from build123d import *

# Parameters (mm, degrees)
F0_W      = 5
F0_H      = 37.2
F0_W_2    = 20
F0_H_2    = 20
F0_W_3    = 23.5
F0_H_3    = 32.2
F0_R      = 10
F1_DEPTH  = 5
F2_DEPTH  = 5.7
F3_DEPTH  = 7
F4_W      = 23.5
F4_H      = 32.2
F4_R      = 10
F5_DEPTH  = 43
F6_R      = 5
F7_SIZE   = 2
F8_SIZE   = 1
F9_SIZE   = 1
F10_SIZE  = 1
F11_R     = 2
F12_R     = 3.3
F13_DEPTH = 3.2
F14_SIZE  = 0.5


with BuildPart() as f1:
    # F0 (on Top) → F1 (new body)
    with BuildSketch(Plane.XY):
        with Locations((-53, 29.4)):
            Rectangle(F0_W, F0_H)
        Polygon((-50.5, 48), (-50.5, 10.8), (-11.75, 10.8), (-11.75, 43), (11.75, 43), (11.75, 10.8), (50.5, 10.8), (50.5, 48), (5, 48), (-5, 48), align=None)
        with Locations((-30.5, 29.4)):
            Rectangle(F0_W_2, F0_H_2, mode=Mode.SUBTRACT)
        with Locations((30.5, 29.4)):
            Rectangle(F0_W_2, F0_H_2, mode=Mode.SUBTRACT)
        with Locations((0, 26.9)):
            Rectangle(F0_W_3, F0_H_3)
        with Locations((0, 26.1)):
            Circle(F0_R, mode=Mode.SUBTRACT)
        with Locations((53, 29.4)):
            Rectangle(F0_W, F0_H)
    extrude(amount=F1_DEPTH)

    # F0 (on Top) → F2 (join)
    with BuildSketch(Plane.XY):
        with Locations((-53, 29.4)):
            Rectangle(F0_W, F0_H)
        with Locations((53, 29.4)):
            Rectangle(F0_W, F0_H)
    extrude(amount=-F2_DEPTH)

    # F0 (on Top) → F3 (join)
    with BuildSketch(Plane.XY):
        with Locations((0, 26.9)):
            Rectangle(F0_W_3, F0_H_3)
        with Locations((0, 26.1)):
            Circle(F0_R, mode=Mode.SUBTRACT)
    extrude(amount=-F3_DEPTH)

    # F4 (on face) → F5 (join)
    with BuildSketch(Plane(origin=(0, 0, -7), x_dir=(1, 0, 0), z_dir=(0, 0, -1))):
        with Locations((0, -26.9)):
            Rectangle(F4_W, F4_H)
        with Locations((0, -26.1)):
            Circle(F4_R, mode=Mode.SUBTRACT)
        with Locations((0, -26.1)):
            Circle(F4_R)
    extrude(amount=F5_DEPTH)

    # F6
    f6_edges = [f1.edges().sort_by_distance(p)[0] for p in [
        (20.5, 39.4, 2.5),
        (40.5, 39.4, 2.5),
        (20.5, 19.4, 2.5),
        (40.5, 19.4, 2.5),
        (-20.5, 39.4, 2.5),
        (-40.5, 39.4, 2.5),
        (-40.5, 19.4, 2.5),
        (-20.5, 19.4, 2.5),
    ]]
    fillet(f6_edges, radius=F6_R)

    # F7
    f7_edges = [f1.edges().sort_by_distance(p)[0] for p in [
        (0, 10.8, -50),
        (-11.75, 26.9, -50),
        (0, 43, -50),
        (11.75, 26.9, -50),
    ]]
    chamfer(f7_edges, length=F7_SIZE)

    # F8
    f8_edges = [f1.edges().sort_by_distance(p)[0] for p in [
        (55.5, 29.4, -5.7),
        (53, 48, -5.7),
        (50.5, 29.4, -5.7),
        (53, 10.8, -5.7),
        (-53, 10.8, -5.7),
        (-50.5, 29.4, -5.7),
        (-53, 48, -5.7),
        (-55.5, 29.4, -5.7),
    ]]
    chamfer(f8_edges, length=F8_SIZE)

    # F9
    f9_edges = [f1.edges().sort_by_distance(p)[0] for p in [
        (-10, 26.1, 5),
        (20.5, 29.4, 5),
        (21.964466, 20.864466, 5),
        (21.964466, 37.935534, 5),
        (30.5, 19.4, 5),
        (30.5, 39.4, 5),
        (39.035534, 20.864466, 5),
        (39.035534, 37.935534, 5),
        (40.5, 29.4, 5),
        (0, 10.8, 5),
        (55.5, 29.4, 5),
        (0, 48, 5),
        (-55.5, 29.4, 5),
        (-40.5, 29.4, 5),
        (-39.035534, 20.864466, 5),
        (-39.035534, 37.935534, 5),
        (-30.5, 19.4, 5),
        (-30.5, 39.4, 5),
        (-21.964466, 20.864466, 5),
        (-21.964466, 37.935534, 5),
        (-20.5, 29.4, 5),
    ]]
    chamfer(f9_edges, length=F9_SIZE)

    # F10
    f10_edges = [f1.edges().sort_by_distance(p)[0] for p in [
        (-30.5, 19.4, 0),
        (-20.5, 29.4, 0),
        (-30.5, 39.4, 0),
        (-40.5, 29.4, 0),
        (30.5, 19.4, 0),
        (20.5, 29.4, 0),
        (30.5, 39.4, 0),
        (40.5, 29.4, 0),
        (-39.035534, 20.864466, 0),
        (-39.035534, 37.935534, 0),
        (-21.964466, 20.864466, 0),
        (-21.964466, 37.935534, 0),
        (21.964466, 20.864466, 0),
        (21.964466, 37.935534, 0),
        (39.035534, 20.864466, 0),
        (39.035534, 37.935534, 0),
    ]]
    chamfer(f10_edges, length=F10_SIZE)

    # F11
    f11_edges = [f1.edges().sort_by_distance(p)[0] for p in [
        (-11.75, 43, -24),
        (11.75, 43, -24),
    ]]
    fillet(f11_edges, radius=F11_R)

    # F12 (on face) → F13 (cut)
    with BuildSketch(Plane.XY):
        with Locations((-46, 43)):
            Circle(F12_R)
        with Locations((46, 15.8)):
            Circle(F12_R)
    extrude(amount=F13_DEPTH, mode=Mode.SUBTRACT)

    # F14
    f14_edges = [f1.edges().sort_by_distance(p)[0] for p in [
        (-49.3, 43, 0),
        (42.7, 15.8, 0),
    ]]
    chamfer(f14_edges, length=F14_SIZE)


solid = f1.part
Source: CAD feature listing. Evaluate the final solid. Frame: model axes, mm. A direction names the side the tool comes from. Round coordinates to 2 decimals unless told otherwise and drop trailing zeros. Loops run counter-clockwise (first coordinate to the right, second up) from the corner with the lowest first, then second, coordinate; pieces in that order, holes last.
Q1. Section A-A, the plane x = -31. Return loops of the section in (y, z), plus the area to 3 significant figures.
Q2. First-contact query: P1, Ø10, axis at x = -0.5, z = -19.5, coming from the +Y side; P2, Ø12, axis at x = 0, y = 26.1, coming from the +Z side; P3, Ø3, axis at x = -34.5, y = 36, coming from the +Z side; P4, Ø9, axis at y = 25.5, z = -13.5, coming from the +X side. Flat tips, straight axial feed; report the tip coordinate or a pass-through.
Q3. Ray query, line 1 (Y direction, x = 0, z = -1); line 2 (Y direction, x = 46, z = 1); line 3 (Z direction, x = -42, y = 28). Return the intervals inside material, ascending.
Q4. Section D-D, the plane y = 26.1. State how many separate pieces and enclosed holes the cut face has, plus the area to 4 significant figures.
Q5. Mould query, pull axis X, two halves, no side actions, for faces 4 (the face through (-21.93, 20.9, 2.52)), 5 (the face through (21.732, 20.714, 0.729)), 6 (the face through (-1, 48, 3)), 7 (the face through (10.74, 26.83, -49.01)). Classes: pulls with the +X half, pulls with the -X half, needs draft (parallel to the pull), parting line crosses it, or undercut.
Q6. Section B-B, the plane z = -35. Return loops of the section in (x, y).
Q7. Access query for faces 1 (the face through (-39.186, 20.632, 4.271)), 2 (the face through (-39.07, 20.9, 2.52)), 3 (the face through (-48.43, 45.23, 1.83)). Directions: +Z, -Z, +X, -X, +Y, -Y. A direction counts if a zero-diameter tool reaches every point of the face in a straight line with its end or side. Return the directions, or none.
Q8. Section C-C, the plane x = 0. Return loops of the section in (y, z), plus the area to 3 significant figures.
Solutions:
1. outline: (10.8, 0) - (18.4, 0) - (19.4, 1) - (19.4, 4) - (18.4, 5) - (11.8, 5) - (10.8, 4) - close; (39.4, 1) - (40.4, 0) - (48, 0) - (48, 4) - (47, 5) - (40.4, 5) - (39.4, 4) - close
1. area: 83.0 mm2
2. P1: stops at y = 43
2. P2: stops at z = -7
2. P3: passes through
2. P4: stops at x = 11.75
3. line 1: y = 10.8 to 16.1, 36.1 to 43
3. line 2: y = 10.8 to 12.5, 19.1 to 48
3. line 3: z = 0 to 5
4. separate pieces: 3
4. enclosed holes: 0
4. area: 1,335 mm2
5. face 4: undercut
5. face 5: undercut
5. face 6: needs draft
5. face 7: pulls with the +X half
6. outline: (-11.75, 10.8) - (11.75, 10.8) - (11.75, 41) arc R2 ccw to (9.75, 43) - (-9.75, 43) arc R2 ccw to (-11.75, 41) - close
7. face 1: +Z
7. face 2: +Z, -Z
7. face 3: -Z
8. outline: (10.8, -48) - (12.8, -50) - (41, -50) - (43, -48) - (43, 0) - (48, 0) - (48, 4) - (47, 5) - (37.1, 5) - (36.1, 4) - (36.1, -7) - (16.1, -7) - (16.1, 4) - (15.1, 5) - (11.8, 5) - (10.8, 4) - close
8. area: 1,550 mm2
